The model under review builds one solid part; all positions refer to its coordinate system, in mm. A direction names the side the tool comes from. Coordinates: 2 decimals unless noted, no trailing zeros. Write each loop counter-clockwise with the first axis right and the second up, starting at its lowest first coordinate (ties: lowest second). Pieces come first, ordered by that corner, then holes.
1) Machinability: for faces 4 (the cylindrical face through (24.636, 13.311, -10.706)), 5 (the flat face through (-17.4, -1, 0)), 6 (the flat face through (21.4, -1, 0)), 7 (the cylindrical face through (23.767, 13.311, 10.22)), which of the approach directions +Z, -Z, +X, -X, +Y, -Y give a long, thin tool a straight path to every point of the face, cutting with its end or side? Answer none if there is none.
2) Add section B-B, the plane z = 2.54. State the section outline as (x, y) points, then the cut area to 3 significant figures.
3) Add section C-C, the plane y = 3.5. State the section outline as (x, z) points (3 decimals).
4) Add section D-D, the plane x = -18.5. State the section outline as (y, z) points.
5) For line 1 (Z direction, x = -22.86, y = 21.75); line 2 (Z direction, x = -22, y = 19); line 3 (X direction, y = 9, z = -8.89), list the stretches that pass through material, from the lowest coordinate up.
6) Add section A-A, the plane x = -3.4. State the section outline as (y, z) points, then the cut area to 3 significant figures.
7) For P1, Ø2, axis at x = -23, z = -9.5, coming from the -Y side; P2, Ø5, axis at x = 15, z = -11, coming from the +Y side; P3, Ø1.3, axis at x = -23, z = 9, coming from the -Y side, all flat-tipped, find the tip position at first contact; note any pin that passes through.
8) Mouldability with a two-part tool opening along X and no side actions: class faces 1 (the cylindrical face through (24.676, 13.311, 10.666)), 2 (the flat face through (2, -1.5, 0)), 3 (the flat face through (-23, 27, 9)) as released by +X, released by -X, zero draft, split by the parting line, or undercut.
Autodesk Inventor part; units mm, degrees
ref_plane "YZ Plane" through (0, 0, 0) normal (1, 0, 0) x (0, 1, 0)
ref_plane "XZ Plane" through (0, 0, 0) normal (0, 1, 0) x (-1, 0, 0)
ref_plane "XY Plane" through (0, 0, 0) normal (0, 0, 1) x (1, 0, 0)
sketch "Sketch1" plane through (0, 0, 0) normal (0, 1, 0) x (-1, 0, 0)
  line L0 (22.86, 11.43) -> (-22.86, 11.43)
  line L1 (-25.4, 8.89) -> (-25.4, -8.89)
  line L2 (-22.86, -11.43) -> (22.86, -11.43)
  line L3 (25.4, -8.89) -> (25.4, 8.89)
  line L4 (25.4, 11.43) -> (-25.4, -11.43) construction
  line L5 (-25.4, 11.43) -> (25.4, -11.43) construction
  circle A0 centre (22.86, 8.89) radius 1.27
  circle A1 centre (22.86, -8.89) radius 1.27
  circle A2 centre (-22.86, 9.525) radius 1.143
  circle A3 centre (-22.86, -9.525) radius 1.143
  arc A4 (25.4, 8.89) -> (22.86, 11.43) centre (22.86, 8.89) ccw
  arc A5 (22.86, -11.43) -> (25.4, -8.89) centre (22.86, -8.89) ccw
  arc A6 (-22.86, 11.43) -> (-25.4, 8.89) centre (-22.86, 8.89) ccw
  arc A7 (-25.4, -8.89) -> (-22.86, -11.43) centre (-22.86, -8.89) ccw
  point P0 (0, 0)
  dimension "d0" = 50.8
  dimension "d1" = 22.86
  dimension "d2" = 2.54
  dimension "d3" = 2.54
  dimension "d4" = 2.286
  dimension "d5" = 2.286
  dimension "d6" = 17.78
  dimension "d7" = 19.05
  dimension "d9" = 8.89
  dimension "d10" = 2.54
  dimension "d11" = 2.54
  dimension "d12" = 9.525
  dimension "d13" = 2.54
  dimension "d14" = 2.54
  dimension "d15" = 2.54
extrude "Extrusion1" add sketch "Sketch1" along normal blind 29
sketch "Sketch8" plane through (0, 29, 0) normal (0, 1, 0) x (1, 0, 0)
  circle A0 centre (-3.4, -2.54) radius 3.75
  line L0 (-25.4, 8.89) -> (-25.4, -8.89)
  point P0 (0, 0)
  dimension "d62" = 7.5
  dimension "d63" = 2.54
  dimension "d64" = 22
extrude "Extrusion8" add sketch "Sketch8" along normal blind 15
sketch "Sketch9" plane through (0, 0, 0) normal (0, -1, 0) x (1, 0, 0)
  line L0 (-17.4, 8.93) -> (21.4, 8.93)
  line L1 (21.4, 8.93) -> (21.4, -8.93)
  line L2 (21.4, -8.93) -> (-17.4, -8.93)
  line L3 (-17.4, -8.93) -> (-17.4, 8.93)
  line L4 (-25.4, -8.89) -> (-25.4, 8.89)
  line L5 (25.4, 8.89) -> (25.4, -8.89)
  line L6 (-22.86, 11.43) -> (22.86, 11.43)
  line L7 (22.86, -11.43) -> (-22.86, -11.43)
  point P0 (0, 0)
  dimension "d67" = 8
  dimension "d68" = 4
  dimension "d69" = 2.5
  dimension "d70" = 2.5
extrude "Extrusion9" add sketch "Sketch9" along normal blind 1.5
sketch "Sketch10" plane through (0, 29, 0) normal (0, 1, 0) x (1, 0, 0)
  line L0 (25.4, 14.43) -> (-25.4, 14.43)
  line L1 (-25.4, 14.43) -> (-25.4, -16.43)
  line L2 (-25.4, -16.43) -> (25.4, -16.43)
  line L3 (25.4, -16.43) -> (25.4, 14.43)
  line L4 (25.4, -8.89) -> (25.4, 8.89)
  line L5 (-25.4, 8.89) -> (-25.4, -8.89)
  line L6 (-22.86, -11.43) -> (22.86, -11.43)
  line L7 (22.86, 11.43) -> (-22.86, 11.43)
  point P0 (0, 0)
  point P1 (25.4, 0)
  point P2 (-25.4, -1)
  dimension "d73" = 5
  dimension "d74" = 3
extrude "Extrusion10" add sketch "Sketch10" against normal blind 2
ref_plane "Work Plane1" through (2, 0, -8.93) normal (-1, 0, 0) x (0, 0, 1)
properties part number "ESP8266 Feather"
Geometry results:
1. face 4: -Z, +X, -Y
1. face 5: +Z, -Z, -X, -Y
1. face 6: +Z, -Z, +X, -Y
1. face 7: -Y
2. outline: (-25.4, 0) - (-17.4, 0) - (-17.4, -1.5) - (21.4, -1.5) - (21.4, 0) - (25.4, 0) - (25.4, 29) - (0.35, 29) - (0.35, 44) - (-7.15, 44) - (-7.15, 29) - (-25.4, 29) - close
2. area: 1,640 mm2
3. outline: (-25.4, -8.89) arc R2.54 ccw to (-22.86, -11.43) - (22.86, -11.43) arc R2.54 ccw to (25.4, -8.89) - (25.4, 8.89) arc R2.54 ccw to (22.86, 11.43) - (-22.86, 11.43) arc R2.54 ccw to (-25.4, 8.89) - close; hole circle Ø2.54 at (-22.86, -8.89); hole circle Ø2.54 at (-22.86, 8.89); hole circle Ø2.286 at (22.86, -9.525); hole circle Ø2.286 at (22.86, 9.525)
4. outline: (0, -11.43) - (27, -11.43) - (27, -14.43) - (29, -14.43) - (29, 16.43) - (27, 16.43) - (27, 11.43) - (0, 11.43) - close
5. line 1: z = -11.43 to -10.16, -7.62 to 7.62, 10.16 to 11.43
5. line 2: z = -11.43 to -9.82, -7.96 to 7.96, 9.82 to 11.43
5. line 3: x = -25.4 to -24.13, -21.59 to 21.91, 23.81 to 25.4
6. outline: (-1.5, -8.93) - (0, -8.93) - (0, -11.43) - (27, -11.43) - (27, -14.43) - (29, -14.43) - (29, -1.21) - (44, -1.21) - (44, 6.29) - (29, 6.29) - (29, 16.43) - (27, 16.43) - (27, 11.43) - (0, 11.43) - (0, 8.93) - (-1.5, 8.93) - close
6. area: 818 mm2
7. P1: stops at y = 0
7. P2: stops at y = 29
7. P3: stops at y = 27
8. face 1: released by +X
8. face 2: zero draft
8. face 3: undercut
